Source: CAD feature listing. Evaluate the final solid. Frame: model axes, mm. Coordinates: 2 decimals unless noted, no trailing zeros. Order: outer loops, then holes, each group sorted by start corner. A loop starts at its lowest first (then second) coordinate and runs counter-clockwise, first axis right, second up. Notation, with made-up numbers: (53.5, 44.5) - (80.5, 44.5) arc R20 cw to (80.5, 55.5) - close; hole circle Ø2 at (-30.5, 57.5). An arc over 180 degrees is marked (long way). One line per question, with ' | ' between items.
from build123d import *

# Parameters (mm, degrees)
ELEVATOR_AXLE_BEARING_R = 7.030128061
ELEVATOR_AXLE_BEARING_W = 6.35
ELEVATOR_AXLE_BEARING_H = 6.35
BOSS_EXTRUDE1_DEPTH     = 6.35


with BuildPart() as part:
    # Elevator Axle Bearing → Boss-Extrude1 (new body)
    with BuildSketch(Plane(origin=(0, 0, 0), x_dir=(1, 0, 0), z_dir=(0, 1, 0))):
        with Locations(Location((0, 0, 0), (0, 0, 270))):
            Circle(ELEVATOR_AXLE_BEARING_R)
        Rectangle(ELEVATOR_AXLE_BEARING_W, ELEVATOR_AXLE_BEARING_H, mode=Mode.SUBTRACT)
    extrude(amount=BOSS_EXTRUDE1_DEPTH)


solid = part.part
(1) Cut plane B-B (z = 0). Return the cut outline in (x, y) (3 decimals).
Taken from the geometry:
outline: (-7.03, 0) - (-3.175, 0) - (-3.175, 6.35) - (-7.03, 6.35) - close; (3.175, 0) - (7.03, 0) - (7.03, 6.35) - (3.175, 6.35) - close
(2) Material intervals for L1, parallel to Z at x = 1, y = 5.25 (3 decimals); L2, parallel to Z at x = 2.5, y = 3.25 (3 decimals); L3, parallel to X at y = 3.25, z = 2.75 (3 decimals), sorted ascending. Write a range as from..to.
Taken from the geometry:
L1: z = -6.959..-3.175, 3.175..6.959 | L2: z = -6.571..-3.175, 3.175..6.571 | L3: x = -6.47..-3.175, 3.175..6.47
(3) Cut plane D-D (z = -5). Return the cut outline in (x, y), and give its area (3 significant figures).
Taken from the geometry:
outline: (-4.94, 0) - (4.94, 0) - (4.94, 6.35) - (-4.94, 6.35) - close | area: 62.8 mm²
(4) Cut plane A-A (x = 0.75). Return the cut outline in (y, z) (3 decimals).
Taken from the geometry:
outline: (0, -6.99) - (6.35, -6.99) - (6.35, -3.175) - (0, -3.175) - close; (0, 3.175) - (6.35, 3.175) - (6.35, 6.99) - (0, 6.99) - close
(5) Pull-direction query (Z, two-part tool) for faces 1 (the flat face through (-3.175, 3, 0)), 2 (the cylindrical face through (6.97, 3.13, -0.92)); classes: pulls with the +Z half, pulls with the -Z half, needs draft (parallel to the pull), parting line crosses it, or undercut.
Taken from the geometry:
face 1: undercut | face 2: parting line crosses it
(6) Cut plane C-C (y = 4.25). Return the cut outline in (x, z) (3 decimals).
Taken from the geometry:
outline: circle Ø14.06 at (0, 0); hole (-3.175, -3.175) - (3.175, -3.175) - (3.175, 3.175) - (-3.175, 3.175) - close
